Drawing for the job (mm, zero at the part's lowest x, y, z). A direction names the side the tool comes from. Coordinates: 2 decimals unless noted, no trailing zeros. Order: outer loops, then holes, each group sorted by start corner. A loop starts at its lowest first (then second) coordinate and runs counter-clockwise, first axis right, second up. Notation, with made-up numbers: (-12.75, 74.25) -> (44.25, 74.25) arc R35 ccw to (44.25, 107.25) -> close; hole circle Ø5 at (64.5, -11.75). An arc over 180 degrees is marked (long way). Write each question's results on one line, items separated by ' | '.
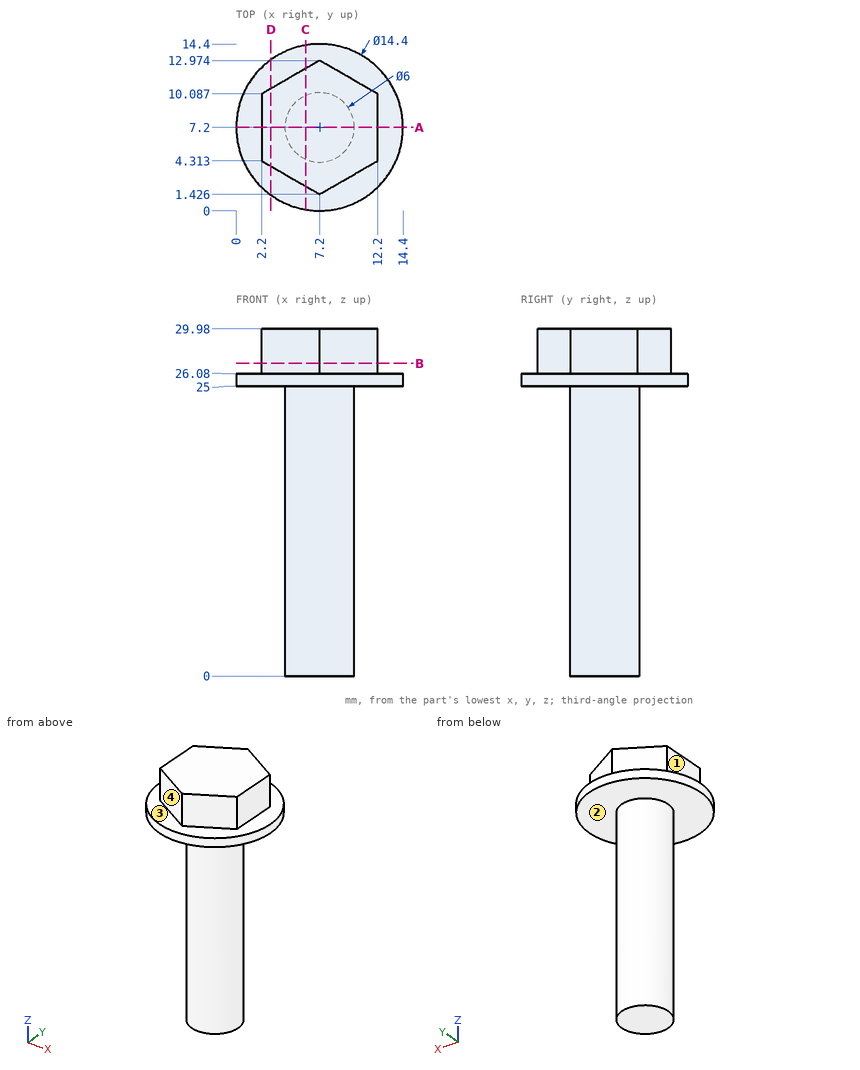
Item 1: Slice it at D-D, the plane x = 3. List the corners of the cut face in (y, z).
Answer:
outline: (1.35, 25) -> (13.05, 25) -> (13.05, 26.08) -> (10.55, 26.08) -> (10.55, 29.98) -> (3.85, 29.98) -> (3.85, 26.08) -> (1.35, 26.08) -> close
Item 2: Tool access for the marked faces 1, 2, 3 and 4: list every direction of +Z, -Z, +X, -X, +Y, -Y with a clear straight run to the whole face (end or side of a thin tool).
Answer:
face 1: +Z, -X, +Y, -Y | face 2: -Z | face 3: +Z | face 4: +Z, -X, -Y
Item 3: Slice it at A-A, the plane y = 7.2. List the corners of the cut face in (x, z).
Answer:
outline: (0, 25) -> (4.2, 25) -> (4.2, 0) -> (10.2, 0) -> (10.2, 25) -> (14.4, 25) -> (14.4, 26.08) -> (12.2, 26.08) -> (12.2, 29.98) -> (2.2, 29.98) -> (2.2, 26.08) -> (0, 26.08) -> close
Item 4: Drill centre lines: line 1 (Z direction, x = 10, y = 3); line 2 (Z direction, x = 3.75, y = 10.75); line 3 (Y direction, x = 7, z = 25.5). Where is each one in solid material? Low to high. Write a range as from..to.
Answer:
line 1: z = 25..26.08 | line 2: z = 25..29.98 | line 3: y = 0..14.4
Item 5: Pin check, flat tips, straight feed: pin 1 (4 mm diameter, centred on x = 12.5, y = 4, fed in from -Z); pin 2 (8 mm diameter, centred on y = 12.5, z = 8.5, fed in from -X); pin 3 (3 mm diameter, centred on y = 6.5, z = 27.5, fed in from -X). Stop position of each tip, or through.
Answer:
pin 1: stops at z = 25 | pin 2: stops at x = 4.5 | pin 3: stops at x = 0
Item 6: Slice it at B-B, the plane z = 27. List the corners of the cut face in (x, y).
Answer:
outline: (2.2, 4.31) -> (7.2, 1.43) -> (12.2, 4.31) -> (12.2, 10.09) -> (7.2, 12.97) -> (2.2, 10.09) -> close
Item 7: Slice it at C-C, the plane x = 6. List the corners of the cut face in (y, z).
Answer:
outline: (0.1, 25) -> (4.45, 25) -> (4.45, 0) -> (9.95, 0) -> (9.95, 25) -> (14.3, 25) -> (14.3, 26.08) -> (12.28, 26.08) -> (12.28, 29.98) -> (2.12, 29.98) -> (2.12, 26.08) -> (0.1, 26.08) -> close
